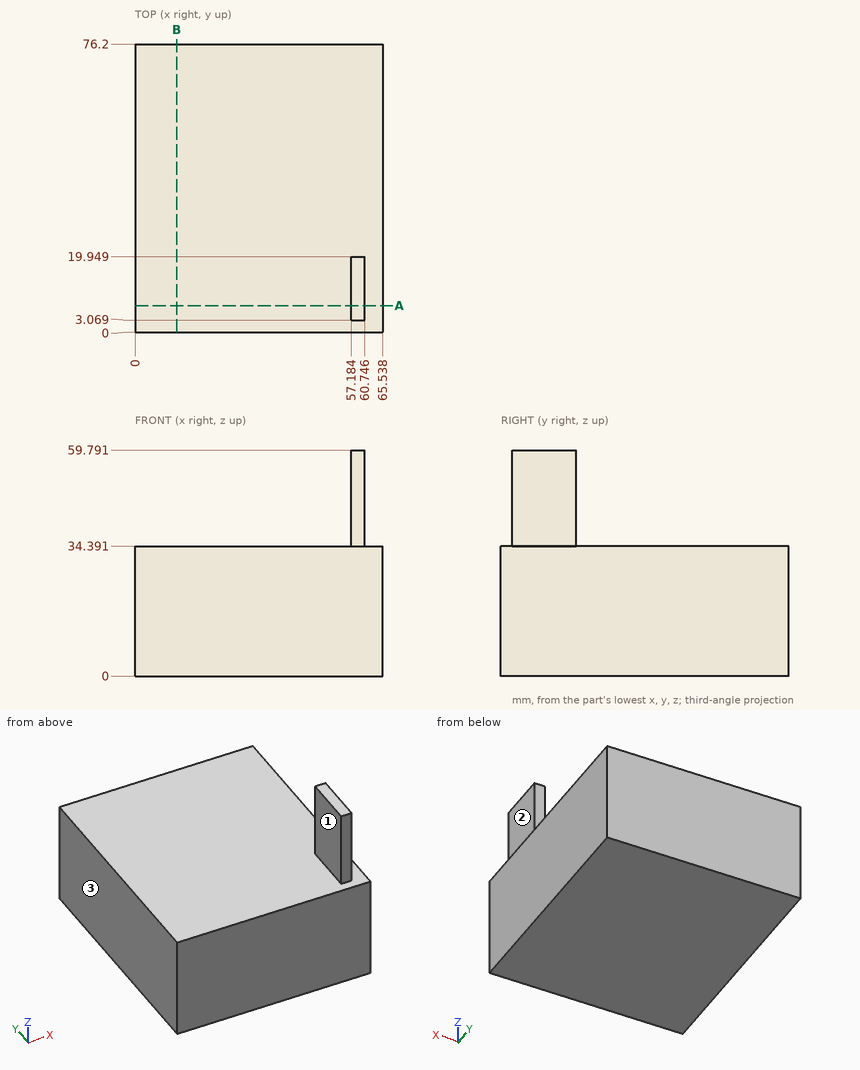
Verification items for this drawing (mm, ordinates from the low corner). A direction names the side the tool comes from. Coordinates: 2 decimals unless noted, no trailing zeros. Loops run counter-clockwise (first coordinate to the right, second up) from the corner with the lowest first, then second, coordinate; pieces in that order, holes last.
Item 1: Sectioned sample at B-B, the plane x = 11. Record the boundary of the cut face in (y, z).
Item 2: Sectioned sample at A-A, the plane y = 7. Record the boundary of the cut face in (x, z) (1 decimal).
Item 3: Go/stop test with flat-tipped pins: pin 1 Ø10 at (x, z) = (40.5, 24.5) entering from -Y; pin 2 Ø1.8 at (x, z) = (58, 49.5) entering from +Y; pin 3 Ø18.5 at (y, z) = (13.5, 44) entering from -X; pin 4 Ø8 at (x, y) = (40.5, 20) entering from +Z. Record where each tip stops, or that it passes through.
Item 4: Thickness scan on line 1 (Z direction, x = 38.5, y = 25). Record the ranges inside material, lowest first.
Item 5: Access from +Z, -Z, +X, -X, +Y, -Y to the whole of each face (thin tool, end or side, straight path). Record for the marked faces 1, 2 and 3.
Check result:
1. outline: (0, 0) - (76.2, 0) - (76.2, 34.39) - (0, 34.39) - close
2. outline: (0, 0) - (65.5, 0) - (65.5, 34.4) - (60.7, 34.4) - (60.7, 59.8) - (57.2, 59.8) - (57.2, 34.4) - (0, 34.4) - close
3. pin 1: stops at y = 0
3. pin 2: stops at y = 19.95
3. pin 3: stops at x = 57.18
3. pin 4: stops at z = 34.39
4. line 1: z = 0 to 34.39
5. face 1: +Z, -X, +Y, -Y
5. face 2: +Z, +X, +Y, -Y
5. face 3: +Z, -Z, -X, +Y, -Y
